The model under review builds one solid part; all positions refer to its coordinate system, in mm. A direction names the side the tool comes from. Round coordinates to 2 decimals unless told otherwise and drop trailing zeros. Write each loop counter-clockwise with the first axis right and the second up, starting at its lowest first coordinate (ties: lowest second). Pieces come first, ordered by that corner, then holes. Notation, with made-up numbers: (-1.5, 68) -> (33.5, 68) arc R16 ccw to (33.5, 77) -> close; hole circle Ø10 at (56.5, -13.5). An arc over 180 degrees is marked (long way). Return JSON: item names as keys, results as strings. Group by question number.
1. Take a section at A-A, the plane y = 2.3. Write out the cut boundary in (x, z).
2. Take a section at D-D, the plane z = 1.5. Write out the cut boundary in (x, y), then the cut area to 3 significant figures.
3. Tool access review of faces 1 (the flat face through (-8.981, 1, -1)), 2 (the flat face through (5, 1.6, 3)): name each direction out of +Z, -Z, +X, -X, +Y, -Y from which nothing blocks a thin tool from reaching the whole face with its end or side.
4. For line 1 along Z through (x, y) = (11, 2.3); line 2 along X through (y, z) = (1.85, -4.5); line 3 along X through (y, z) = (0.7, -0.5), list the stretches that pass through material, from the lowest coordinate up. Write a range as from..to.
5. Take a section at B-B, the plane x = 17. Write out the cut boundary in (y, z).
6. Clearance check with flat-ended pins moving along their axes: P1, Ø8, axis at x = -5.5, z = 1.5, coming from the +Y side; P2, Ø3, axis at x = -4.98, z = -0.92, coming from the +Y side. State where each tip first meets the part, or that it passes through.
7. Mouldability with a two-part tool opening along X and no side actions: class faces 3 (the flat face through (5, 0, 1)), 4 (the flat face through (5.082, 1.093, 1.316)), 5 (the flat face through (19.019, 1, -1)) as pulls with the +X half, pulls with the -X half, needs draft (parallel to the pull), parting line crosses it, or undercut.
8. Take a section at C-C, the plane z = -6.75. Write out the cut boundary in (x, y), then the cut area to 3 significant figures.
Autodesk Inventor part; units mm, degrees
ref_plane "YZ Plane" through (0, 0, 0) normal (1, 0, 0) x (0, 1, 0)
ref_plane "XZ Plane" through (0, 0, 0) normal (0, 1, 0) x (-1, 0, 0)
ref_plane "XY Plane" through (0, 0, 0) normal (0, 0, 1) x (1, 0, 0)
sketch "Эскиз1" plane through (0, 0, 0) normal (0, 1, 0) x (-1, 0, 0)
  line L0 (8.9811, 8.3302) -> (-19.0189, 8.3302)
  line L1 (-19.0189, 8.3302) -> (-19.0189, -10.1698)
  line L2 (-19.0189, -10.1698) -> (8.9811, -10.1698)
  line L3 (8.9811, -10.1698) -> (8.9811, 8.3302)
  point P0 (0, 0)
  dimension "d0" = 28
  dimension "d1" = 18.5
extrude "Выдавливание1" add sketch "Эскиз1" along normal blind 1.6
sketch "Эскиз2" plane through (0, 1.6, 0) normal (0, 1, 0) x (1, 0, 0)
  line L0 (-8.9811, -8.3302) -> (19.0189, -8.3302)
  line L1 (19.0189, -8.3302) -> (19.0189, 10.1698)
  line L2 (19.0189, 10.1698) -> (-8.9811, 10.1698)
  line L3 (-8.9811, 10.1698) -> (-8.9811, -8.3302)
  line L4 (-7.4811, -6.8302) -> (17.5189, -6.8302)
  line L5 (17.5189, -6.8302) -> (17.5189, 8.6698)
  line L6 (17.5189, 8.6698) -> (-7.4811, 8.6698)
  line L7 (-7.4811, 8.6698) -> (-7.4811, -6.8302)
  point P0 (0, 0)
  dimension "d4" = 1.5
extrude "Выдавливание2" add sketch "Эскиз2" along normal blind 1
sketch "Эскиз3" plane through (0, 1.6, 0) normal (0, 1, 0) x (1, 0, 0)
  line L0 (2.5189, -0.3302) -> (7.5189, -0.3302)
  line L1 (7.5189, -0.3302) -> (7.5189, 2.1698)
  line L2 (7.5189, 2.1698) -> (2.5189, 2.1698)
  line L3 (2.5189, 2.1698) -> (2.5189, -0.3302)
  line L4 (-7.4811, 8.6698) -> (-7.4811, -6.8302) construction
  line L5 (-7.4811, -6.8302) -> (17.5189, -6.8302) construction
  line L6 (17.5189, -6.8302) -> (17.5189, 8.6698) construction
  line L7 (17.5189, 8.6698) -> (-7.4811, 8.6698) construction
  line L8 (5.0189, -0.3302) -> (5.0189, -6.8302) construction
  line L9 (5.0189, 2.1698) -> (5.0189, 8.6698) construction
  line L10 (-7.4811, 0.9198) -> (2.5189, 0.9198) construction
  line L11 (7.5189, 0.9198) -> (17.5189, 0.9198) construction
  point P0 (0, 0)
  dimension "d7" = 5
  dimension "d8" = 2.5
extrude "Выдавливание3" cut sketch "Эскиз3" against normal through all
chamfer "Фаска1" distance 2 distance2 1 1 edges at (5.0189, 1.6, -2.1698) measured on face at (5.8522, 1.6, -6.5031)
chamfer "Фаска2" distance 2 distance2 1 1 edges at (2.5189, 1.6, -0.9198) measured on face at (5.8522, 1.6, 4.6635)
chamfer "Фаска3" distance 2 distance2 1 1 edges at (5.0189, 1.6, 0.3302) measured on face at (5.8522, 1.6, 4.6635)
chamfer "Фаска4" distance 2 distance2 1 1 edges at (7.5189, 1.6, -0.9198) measured on face at (14.1855, 1.6, -0.5031)
sketch "Эскиз4" plane through (0, 1.6, 0) normal (0, 1, 0) x (1, 0, 0)
  line L0 (-7.4811, 8.6698) -> (17.5189, 8.6698)
  line L1 (-4.9811, 0.9198) -> (-7.4811, 0.9198) construction
  line L2 (15.0189, 0.9198) -> (17.5189, 0.9198) construction
  line L3 (-7.4811, -6.8302) -> (-7.4811, 8.6698) construction
  line L4 (17.5189, 8.6698) -> (17.5189, -6.8302) construction
  point P0 (0, 0)
  dimension "d24" = 20
hole "Отверстие1" at (15.0189, 1.6, -0.9198) at (-4.9811, 1.6, -0.9198) direction (0, -1, 0) diameter 2.8 end through all
properties part number "SensorShield"
Output:
{
 "1": {"outline": "(-8.98, -10.17) -> (19.02, -10.17) -> (19.02, 8.33) -> (-8.98, 8.33) -> close; hole (-7.48, -8.67) -> (17.52, -8.67) -> (17.52, 6.83) -> (-7.48, 6.83) -> close"},
 "2": {"outline": "(-8.98, 0) -> (19.02, 0) -> (19.02, 2.6) -> (17.52, 2.6) -> (17.52, 1.6) -> (9.52, 1.6) -> (8.69, 1.18) -> (1.35, 1.18) -> (0.52, 1.6) -> (-7.48, 1.6) -> (-7.48, 2.6) -> (-8.98, 2.6) -> close", "area": "44.4 mm^2"},
 "3": {"face 1": "+Z, -Z, -X, +Y, -Y", "face 2": "+Y"},
 "4": {"line 1": "z = -10.17..-8.67, 6.83..8.33", "line 2": "x = -8.98..-7.48, 17.52..19.02", "line 3": "x = -8.98..-6.32, -3.65..2.32, 7.72..13.68, 16.35..19.02"},
 "5": {"outline": "(0, -10.17) -> (2.6, -10.17) -> (2.6, -8.67) -> (1.6, -8.67) -> (1.6, 6.83) -> (2.6, 6.83) -> (2.6, 8.33) -> (0, 8.33) -> close"},
 "6": {"P1": "stops at y = 2.6", "P2": "stops at y = 1.6"},
 "7": {"face 3": "needs draft", "face 4": "undercut", "face 5": "pulls with the +X half"},
 "8": {"outline": "(-8.98, 0) -> (19.02, 0) -> (19.02, 2.6) -> (17.52, 2.6) -> (17.52, 1.6) -> (-7.48, 1.6) -> (-7.48, 2.6) -> (-8.98, 2.6) -> close", "area": "47.8 mm^2"}
}
